Input: part model. Units: mm. Frame: model coordinates. Face numbers are marked on the shaded views. A direction names the side the tool comes from. Give positions to 0.01 mm unless a question says otherwise; leave off trailing zeros. Loops run counter-clockwise (first coordinate to the right, second up) from the corner with the lowest first, then second, coordinate; pieces in that order, holes last. Notation, with made-up numbers: (-16.5, -6) -> (23.5, -6) arc R18 cw to (23.5, 5) -> close; hole circle Ø1 at (-12.5, -33.5). An arc over 180 degrees is marked (long way). Answer as a JSON object with one key per item and string values.
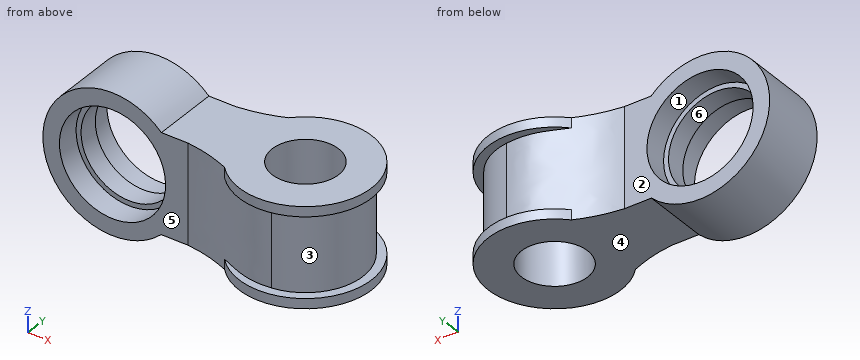
```python
from build123d import *

# Parameters (mm, degrees)
SKETCH1_R                = 20
BOSS_EXTRUDE1_DEPTH      = 3
BOSS_EXTRUDE2_DEPTH      = 30
BOSS_EXTRUDE3_START      = -3
SKETCH3_R                = 20
BOSS_EXTRUDE3_DEPTH      = 3
SKETCH4_R                = 10
CUT_EXTRUDE1_DEPTH       = 43
SKETCH6_R                = 21
SKETCH6_R_2              = 16
BOSS_EXTRUDE4_DEPTH      = 20
SKETCH7_R                = 16
CUT_EXTRUDE2_DEPTH       = 20
BOSS_EXTRUDE5_DEPTH      = 3
BOSS_EXTRUDE5_DEPTH_BACK = 3
SKETCH8_R                = 21
SKETCH8_R_2              = 14.5


with BuildPart() as part:
    # Sketch1 → Boss-Extrude1 (new body)
    with BuildSketch(Plane.XY):
        Circle(SKETCH1_R)
    extrude(amount=BOSS_EXTRUDE1_DEPTH)

    # Sketch2 → Boss-Extrude2 (add)
    with BuildSketch(Plane(origin=(0, 0, 0), x_dir=(-1, 0, 0), z_dir=(0, 0, -1))):
        with BuildLine():
            Line((40, 10), (40, -10))
            Line((40, -10), (28.244450832, -10))
            add(Edge.make_bspline(
                [(28.244450832, -10), (12.990267169, -11.555535356), (9.900933724, -18.719511351), (-2.100622964, -17.258760722)],
                knots=[0, 0, 0, 0, 1, 1, 1, 1], degree=3))
            ThreePointArc((-2.100622964, -17.258760722), (-17.38612776, 0), (-2.100622964, 17.258760722))
            add(Edge.make_bspline(
                [(28.244450832, 10), (12.990267169, 11.555535356), (9.900933724, 18.719511351), (-2.100622964, 17.258760722)],
                knots=[0, 0, 0, 0, 1, 1, 1, 1], degree=3))
            Line((28.244450832, 10), (40, 10))
        make_face()
    extrude(amount=-BOSS_EXTRUDE2_DEPTH)

    # Sketch3 → Boss-Extrude3 (add)
    with BuildSketch(Plane.XY.offset(30).offset(BOSS_EXTRUDE3_START)):
        Circle(SKETCH3_R)
    extrude(amount=BOSS_EXTRUDE3_DEPTH)

    # Sketch4 → Cut-Extrude1 (cut)
    with BuildSketch(Plane(origin=(0, 0, 0), x_dir=(-1, 0, 0), z_dir=(0, 0, -1))):
        Circle(SKETCH4_R)
    extrude(amount=-CUT_EXTRUDE1_DEPTH, mode=Mode.SUBTRACT)

    # Sketch6 → Boss-Extrude4 (add)
    with BuildSketch(Plane(origin=(0, 10, 0), x_dir=(1, 0, 0), z_dir=(0, 1, 0))):
        with Locations((-51, -15.043878404)):
            Circle(SKETCH6_R)
        with Locations((-51, -15.043878404)):
            Circle(SKETCH6_R_2, mode=Mode.SUBTRACT)
    extrude(amount=-BOSS_EXTRUDE4_DEPTH)

    # Sketch7 → Cut-Extrude2 (cut)
    with BuildSketch(Plane(origin=(0, 10, 0), x_dir=(1, 0, 0), z_dir=(0, 1, 0))):
        with Locations(Location((-51, -15.043878404, 0), (0, 0, 180))):
            Circle(SKETCH7_R)
    extrude(amount=-CUT_EXTRUDE2_DEPTH, mode=Mode.SUBTRACT)

    # Sketch8 → Boss-Extrude5 (add, two sides: drawn at the far end of the back side and taken through both)
    with BuildSketch(Plane(origin=(0, 0, 0), x_dir=(1, 0, 0), z_dir=(0, 1, 0)).offset(-BOSS_EXTRUDE5_DEPTH_BACK)):
        with Locations((-51, -15.043878404)):
            Circle(SKETCH8_R)
        with Locations(Location((-51, -15.043878404, 0), (0, 0, 270))):
            Circle(SKETCH8_R_2, mode=Mode.SUBTRACT)
    extrude(amount=BOSS_EXTRUDE5_DEPTH + BOSS_EXTRUDE5_DEPTH_BACK)


solid = part.part
```
Q1. Section C-C, the plane y = -5. Return the cut outline in (x, z), then the cut area to 3 significant figures.
Evaluation:
{"outline": "(-36.35, 0) -> (-8.66, 0) -> (-8.66, 30) -> (-36.26, 30) arc R21 ccw (long way) to start; (8.66, 0) -> (19.36, 0) -> (19.36, 3) -> (16.65, 3) -> (16.65, 27) -> (19.36, 27) -> (19.36, 30) -> (8.66, 30) -> close; hole circle Ø32 at (-51, 15.04)", "area": "1,540 mm2"}
Q2. Section D-D, the plane z = 34.5. Return the cut outline in (x, y), then the cut area to 3 significant figures.
Evaluation:
{"outline": "(-58.9, -10) -> (-43.1, -10) -> (-43.1, 10) -> (-58.9, 10) -> close", "area": "316 mm2"}
Q3. Access query for the marked faces 1, 2 and 3. Directions: +Z, -Z, +X, -X, +Y, -Y. A direction counts if a zero-diameter tool reaches every point of the face in a straight line with its end or side. Return the directions, or none.
Evaluation:
{"face 1": "+Y", "face 2": "+Z, -Z, -X, +Y", "face 3": "+X"}
Q4. Section B-B, the plane x = -51. Return the cut outline in (y, z).
Evaluation:
{"outline": "(-10, -5.96) -> (10, -5.96) -> (10, -0.96) -> (3, -0.96) -> (3, 0.54) -> (-3, 0.54) -> (-3, -0.96) -> (-10, -0.96) -> close; (-10, 31.04) -> (-3, 31.04) -> (-3, 29.54) -> (3, 29.54) -> (3, 31.04) -> (10, 31.04) -> (10, 36.04) -> (-10, 36.04) -> close"}
Q5. Ray query, line 1 along Z through (x, y) = (-51, -7.5); line 2 along X through (y, z) = (-4, 11.5); line 3 along Z through (x, y) = (-24, -5.5). Return the intervals inside material, ascending.
Evaluation:
{"line 1": "z = -5.96 to -0.96, 31.04 to 36.04", "line 2": "x = -71.7 to -66.6, -35.4 to -9.17, 9.17 to 16.92", "line 3": "z = 0 to 30"}
Q6. Draft query along Z for the marked faces 4, 5 and 6. Return one class per face: +Z half, -Z half, draft (parallel to the pull), parting line (faces both ways), or undercut.
Evaluation:
{"face 4": "-Z half", "face 5": "draft", "face 6": "undercut"}
Q7. Pin query (flat end, axial travel): pin 1 (17.5 mm diameter, centred on x = -5, y = -1.5, fed in from +Z); pin 2 (1.5 mm diameter, centred on y = -15.5, z = 24.5, fed in from +X); pin 3 (12 mm diameter, centred on y = 14.5, z = 24.5, fed in from +X). Return the tip coordinate at first contact, or that it passes through.
Evaluation:
{"pin 1": "stops at z = 30", "pin 2": "stops at x = 9.2", "pin 3": "stops at x = 17.84"}
Q8. Section A-A, the plane y = 0. Return the cut outline in (x, z).
Evaluation:
{"outline": "(-36.35, 0) -> (-10, 0) -> (-10, 30) -> (-36.26, 30) arc R21 ccw (long way) to start; (10, 0) -> (20, 0) -> (20, 3) -> (17.39, 3) -> (17.39, 27) -> (20, 27) -> (20, 30) -> (10, 30) -> close; hole circle Ø29 at (-51, 15.04)"}
